The listing builds one solid part. Answer for the finished solid, in the listing's coordinates (mm). Face numbers are marked on the shaded views. A direction names the side the tool comes from. Coordinates: 2 decimals unless noted, no trailing zeros. Order: outer loops, then holes, each group sorted by start corner. A loop starts at its lowest first (then second) coordinate and runs counter-clockwise, first axis right, second up. Notation, with made-up numbers: (26.25, 76) -> (73.25, 76) arc R29 ccw to (73.25, 103) -> close; hole circle Ø9 at (-29, 6.25). An arc over 180 degrees is marked (long way). Write each question's results on one line, items separated by ' | '. Start each with the question number.
(1) Straight lines are drawn through the part: L1, parallel to X at y = 271, z = 3.85; L2, parallel to Y at x = 175, z = 4.25; L3, parallel to Y at x = 121.5, z = 2. For each, find the intervals that lie inside material, in ascending order.
(2) Given pin 1 (11 mm diameter, centred on x = 85, y = 271, fed in from -Z); pin 2 (9 mm diameter, centred on x = 40, y = 271, fed in from +Z); pin 3 (0.5 mm diameter, centred on y = 268.5, z = 4, fed in from -X), each flat-ended and moving along its own axis, determine where each tip first touches the part or whether it passes through.
(3) The part is cut by section A-A, the plane x = 85. Give the vertices of the cut face in (y, z), then the cut area to 3 significant figures.
(4) The part is cut by section C-C, the plane x = 201. Give the vertices of the cut face in (y, z).
(5) A tool of negligible diameter and unlimited length cuts with its end or side. For the marked faces 1, 2 and 3, from which of +Z, -Z, +X, -X, +Y, -Y can it reach the whole face along a straight path? Write none if from no direction.
(6) The part is cut by section B-B, the plane z = 1.75. Give the vertices of the cut face in (x, y), then the cut area to 3 significant figures.
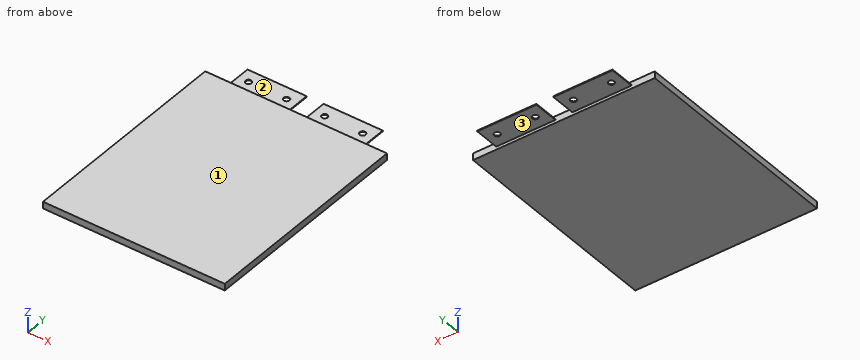
```python
from build123d import *

# Parameters (mm, degrees)
SKETCH2_W           = 215
SKETCH2_H           = 256
BOSS_EXTRUDE1_DEPTH = 8
SKETCH3_W           = 70
SKETCH3_H           = 1
BOSS_EXTRUDE3_DEPTH = 30
CUT_EXTRUDE1_REACH  = 359.829
SKETCH5_R           = 3.5


with BuildPart() as part:
    # Sketch2 → Boss-Extrude1 (new body)
    with BuildSketch(Plane.XY):
        with Locations((107.5, 128)):
            Rectangle(SKETCH2_W, SKETCH2_H)
    extrude(amount=BOSS_EXTRUDE1_DEPTH)

    # Sketch3 → Boss-Extrude3 (add)
    with BuildSketch(Plane(origin=(0, 256, 0), x_dir=(1, 0, 0), z_dir=(0, 1, 0))):
        with Locations((62.5, -4)):
            Rectangle(SKETCH3_W, SKETCH3_H)
        with Locations((152.5, -4)):
            Rectangle(SKETCH3_W, SKETCH3_H)
    extrude(amount=BOSS_EXTRUDE3_DEPTH)

    # Sketch5 → Cut-Extrude1 (cut, up to next)
    with BuildSketch(Plane.XY.offset(4.5), mode=Mode.PRIVATE) as cut_extrude1_sk1:
        with Locations((40, 271)):
            Circle(SKETCH5_R)
    cut_extrude1_tool1 = extrude(cut_extrude1_sk1.sketch, amount=-CUT_EXTRUDE1_REACH, mode=Mode.PRIVATE) & part.part
    # Sketch5 → Cut-Extrude1 (cut, up to next)
    with BuildSketch(Plane.XY.offset(4.5), mode=Mode.PRIVATE) as cut_extrude1_sk2:
        with Locations((85, 271)):
            Circle(SKETCH5_R)
    cut_extrude1_tool2 = extrude(cut_extrude1_sk2.sketch, amount=-CUT_EXTRUDE1_REACH, mode=Mode.PRIVATE) & part.part
    cut_extrude1_1 = cut_extrude1_tool1.solids().sort_by_distance((40, 271, 4.5))[0]
    add(cut_extrude1_1, mode=Mode.SUBTRACT)
    cut_extrude1_2 = cut_extrude1_tool2.solids().sort_by_distance((85, 271, 4.5))[0]
    add(cut_extrude1_2, mode=Mode.SUBTRACT)
    cut_extrude1 = cut_extrude1_1 + cut_extrude1_2  # Cut-Extrude1 as one shape, for the pattern or mirror that repeats it

    # Mirror1: Cut-Extrude1 across plane
    add(cut_extrude1.mirror(Plane(origin=(107.5, 0, 0), x_dir=(0, 0, 1), z_dir=(1, 0, 0))), mode=Mode.SUBTRACT)


solid = part.part
```
Established:
1) L1: x = 27.5 to 36.5, 43.5 to 81.5, 88.5 to 97.5, 117.5 to 126.5, 133.5 to 171.5, 178.5 to 187.5 | L2: y = 0 to 267.5, 274.5 to 286 | L3: y = 0 to 256
2) pin 1: stops at z = 3.5 | pin 2: stops at z = 4.5 | pin 3: stops at x = 27.5
3) outline: (0, 0) -> (256, 0) -> (256, 3.5) -> (267.5, 3.5) -> (267.5, 4.5) -> (256, 4.5) -> (256, 8) -> (0, 8) -> close; (274.5, 3.5) -> (286, 3.5) -> (286, 4.5) -> (274.5, 4.5) -> close | area: 2,070 mm^2
4) outline: (0, 0) -> (256, 0) -> (256, 8) -> (0, 8) -> close
5) face 1: +Z, +X, -X, +Y, -Y | face 2: +Z, +X, -X, +Y | face 3: -Z, +X, -X, +Y
6) outline: (0, 0) -> (215, 0) -> (215, 256) -> (0, 256) -> close | area: 55,000 mm^2
